Autodesk Inventor part; units mm, degrees
ref_plane "Work Plane1" through (30, 0, 0) normal (0, -0.5, 0.866) x (1, 0, 0)
ref_plane "YZ Plane" through (0, 0, 0) normal (1, 0, 0) x (0, 1, 0)
ref_plane "XZ Plane" through (0, 0, 0) normal (0, 1, 0) x (-1, 0, 0)
sketch "Sketch1" plane through (0, 0, 0) normal (0, 0, 1) x (1, 0, 0)
  line L0 (-1.3333, 0) -> (25, 0)
  line L1 (25, 0) -> (25, 3)
  line L2 (25, 3) -> (1.8269, 3)
  line L3 (1.8269, 3) -> (1.2134, 3)
  line L4 (1.2134, 3) -> (0, 3)
  line L5 (0, 3) -> (0, 5)
  line L6 (0, 5) -> (-6, 5)
  line L7 (-6, 5) -> (-6, 2.8868)
  line L8 (-6, 2.8868) -> (-3, 2.8868)
  line L9 (-3, 2.8868) -> (-1.3333, 0)
  line L10 (-12.2, 0) -> (31.2, 0)
  line L11 (0, -1) -> (0, 6)
  line L12 (1.8269, 3) -> (0, 3) construction
  dimension "d0" = 23.1731
  dimension "d1" = 0.6135
  dimension "d2" = 6
  dimension "d3" = 3
  dimension "d4" = 60
  dimension "d5" = 6
  dimension "d6" = 6
  dimension "d7" = 5.7735
  dimension "d8" = 10
  dimension "d19" = 25
revolve "Body" add sketch "Sketch1" angle 360 about axis through (-1.3333, 0, 0) along (1, 0, 0)
sketch "Sketch2" plane through (-6, 0, 0) normal (-1, 0, 0) x (0, 0, 1)
  circle A0 centre (0, 0) radius 2.8868
  line L0 (0, -7) -> (0, 7)
  line L1 (-7, 0) -> (7, 0)
  line L2 (2.8868, 0) -> (1.4434, -2.5)
  line L3 (1.4434, -2.5) -> (-1.4434, -2.5)
  line L4 (-1.4434, -2.5) -> (-2.8868, 0)
  line L5 (-2.8868, 0) -> (-1.4434, 2.5)
  line L6 (-1.4434, 2.5) -> (1.4434, 2.5)
  line L7 (1.4434, 2.5) -> (2.8868, 0)
extrude "Slot" add sketch "Sketch2" against normal up to next contours L7 A0 | A0 L2 | L6 L0 A0 | A0 L0 L3 | L0 L6 A0 | A0 L3 L0 | L4 A0 | A0 L5
fillet "Fillet2" radius 0.6 1 edges at (-6, -5, 0)
thread "Thread"
chamfer "Chamfer1" distance 0.6135 distance2 0.6135 1 edges at (25, -3, 0) measured on face at (25, -0.5681, -0.823)
fillet "Fillet1" radius 0.25 1 edges at (0, -3, 0)
ref_plane "Work Plane1" through (30, 0, 0) normal (0, -0.5, 0.866) x (1, 0, 0)
equation "\"d0\" = GEL"
equation "\"d1\" = GAL"
equation "\"d2\" = KOH"
equation "\"d3\" = INTI"
equation "\"d5\" = GD"
equation "\"d6\" = BDM"
equation "\"d7\" = 1.1547 * SW"
equation "\"d8\" = KOD"
equation "\"d19\" = NLG"
equation "\"d16\" = RR"
equation "\"d12\" = GEL"
equation "\"d14\" = -0.5 * SPD + 0.5 * GD"
equation "\"d15\" = GUL"
equation "\"d29\" = R"
equation "\"GD\" = NND"
equation "\"NLG\" = 25"
equation "\"GEL\" = 23.1731"
equation "\"KOD\" = 10"
equation "\"KOH\" = 6"
equation "\"INTI\" = 3"
equation "\"GAL\" = 0.61345 * PTC"
equation "\"GUL\" = 0.61345 * PTC"
equation "\"BDM\" = NND"
equation "\"SW\" = 5"
equation "\"RR\" = 0.6"
equation "\"SPD\" = 4.7731"
equation "\"d28\" = R"
equation "\"R\" = 0.25"
equation "\"TOA\" = 30deg"
equation "\"THREADDIA\" = 6"
equation "\"PTC\" = 1"
equation "\"NND\" = 6"
equation "\"E0\" = 1.155 * SW"
equation "\"GD1\" = THREADDIA - 1.2269 * PTC"
properties part number "ANSI B18.3.1M - M6x1 x 25, BSHCSM" material "Steel, Mild"
Can you work these out from the model? Positions are in its coordinate system, mm. A direction names the side the tool comes from. Give positions to 0.01 mm unless a question says otherwise; leave off trailing zeros. Order: outer loops, then holes, each group sorted by start corner. A loop starts at its lowest first (then second) coordinate and runs counter-clockwise, first axis right, second up. Notation, with made-up numbers: M 74.25,67 L 113.25,67 A15 cw 113.25,80 Z; hole C 9,26 d10. An arc over 180 degrees is marked long. One line per question, with ' | ' between items.
Item 1: I'm going to push flat-ended pins straight in: pin 1 Ø6 at (x, y) = (13, 2) entering from -Z; pin 2 Ø6 at (x, z) = (5, 2.5) entering from +Y. Where does each tip first touch, or does it pass through?
Answer block:
pin 1: stops at z = -3 | pin 2: stops at y = 3
Item 2: We'd pull the mould along Y, two halves only. Please class faces 1 (the face through (-2.74, -1.08, 4.88)), 2 (the face through (-6, -2, 2)), 3 (the face through (-4.411, 1.233, -2.175)): released by +Y, released by -Y, zero draft, split by the parting line, or undercut.
Answer block:
face 1: split by the parting line | face 2: zero draft | face 3: undercut
Item 3: For faces 4 (the face through (-4, 2.5, 0)), 5 (the face through (12, -3, 0)), 6 (the face through (25, 0, 0)), which set-ups out of +Z, -Z, +X, -X, +Y, -Y let a thin tool reach every point of the face, with its end or its side?
Answer block:
face 4: -X | face 5: +X | face 6: +Z, -Z, +X, +Y, -Y
Item 4: Suppose I cut it at A-A, the plane x = 3.5. Write out the boundary of the cut face in (y, z).
Answer block:
outline: C 0,0 d6
Item 5: Please list where these lines run through material, in increasing order: L1, parallel to X at y = 0.5, z = 4; L2, parallel to Z at x = 1, y = 0; L3, parallel to Y at x = 6, z = -0.25.
Answer block:
L1: x = -6 to 0 | L2: z = -3 to 3 | L3: y = -2.99 to 2.99
